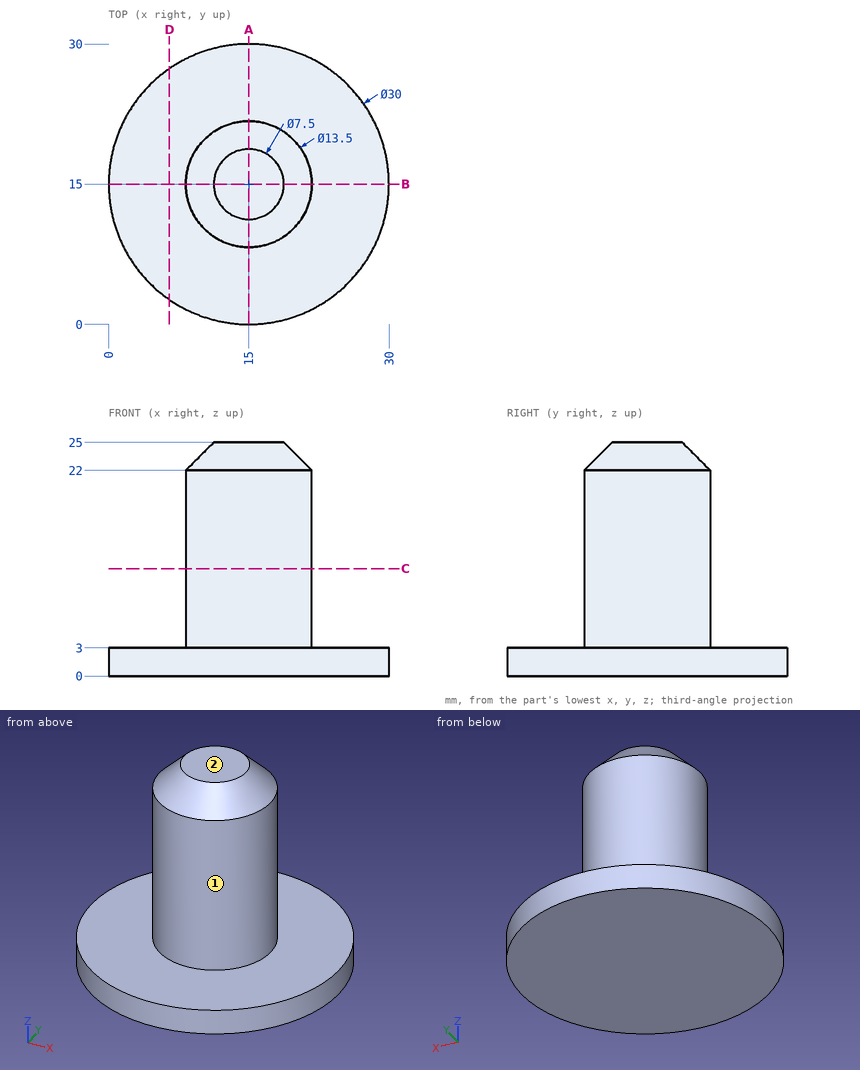
The drawing under review shows one solid part. Ordinate dimensions are in mm from its lowest x, y, z. A direction names the side the tool comes from. Round coordinates to 2 decimals unless told otherwise and drop trailing zeros. Order: outer loops, then holes, each group sorted by start corner. A loop starts at its lowest first (then second) coordinate and runs counter-clockwise, first axis right, second up. Notation, with made-up numbers: (35, -11.75) - (78, -11.75) arc R21 ccw to (78, -1.75) - close; hole circle Ø10 at (-6, 42). An arc over 180 degrees is marked (long way). Return JSON: item names as keys, results as strings.
Q1. Machinability: for the marked faces 1 and 2, which of the approach directions +Z, -Z, +X, -X, +Y, -Y give a long, thin tool a straight path to every point of the face, cutting with its end or side? Answer none if there is none.
Computed values:
{"face 1": "+Z", "face 2": "+Z, +X, -X, +Y, -Y"}
Q2. For pin 1 Ø3 at (x, y) = (24, 21) entering from +Z; pin 2 Ø6 at (y, z) = (6.5, 14.5) entering from -X; pin 3 Ø6 at (y, z) = (8.5, 10) entering from -X, all flat-tipped, find the tip position at first contact; note any pin that passes through.
Computed values:
{"pin 1": "stops at z = 3", "pin 2": "stops at x = 11.09", "pin 3": "stops at x = 9.23"}
Q3. Consider section D-D on x = 6.5. Write out the cut boundary in (y, z), plus the area to 3 significant figures.
Computed values:
{"outline": "(2.64, 0) - (27.36, 0) - (27.36, 3) - (2.64, 3) - close", "area": "74.2 mm2"}
Q4. Consider section C-C on z = 11.5. Write out the cut boundary in (x, y).
Computed values:
{"outline": "circle Ø13.5 at (15, 15)"}
Q5. Consider section A-A on x = 15. Write out the cut boundary in (y, z).
Computed values:
{"outline": "(0, 0) - (30, 0) - (30, 3) - (21.75, 3) - (21.75, 22) - (18.75, 25) - (11.25, 25) - (8.25, 22) - (8.25, 3) - (0, 3) - close"}
Q6. Wall thickness on L1, parallel to Z at x = 17, y = 4.75; L2, parallel to Y at x = 11.75, z = 7; L3, parallel to X at y = 11, z = 2.5: over which ranges is each line inside the solid? List them lowest first. Write a range as [from, to].
Computed values:
{"L1": "z = [0, 3]", "L2": "y = [9.08, 20.92]", "L3": "x = [0.54, 29.46]"}
